from build123d import *

# Parameters (mm, degrees)
F1_DEPTH = 101.6
F2_R     = 5.08
F3_W     = 84.073769
F3_H     = 17.519306
F4_DEPTH = 65.613113


with BuildPart() as f1:
    # F0 (on Right) → F1 (new body)
    with BuildSketch(Plane.YZ):
        Polygon((-46.600301, 33.859685), (-63.820757, 33.859685), (-63.820757, -25.866956), (-42.458672, -25.866956), (-42.458672, -17.365716), (-15.865058, -17.365716), (-15.865058, -26.084935), (1.791356, -26.084935), (1.791356, 3.996365), (-46.600301, 3.996365), align=None)
    extrude(amount=F1_DEPTH)

    # F2
    f2_edges = [f1.edges().sort_by_distance(p)[0] for p in [
        (50.8, -63.820757, 33.859685),
        (50.8, -63.820757, -25.866956),
        (0, -63.820757, 3.996365),
        (101.6, -63.820757, 3.996365),
        (50.8, 1.791356, 3.996365),
        (101.6, -22.404472, 3.996365),
        (0, -22.404472, 3.996365),
        (0, -55.210529, 33.859685),
        (50.8, -46.600301, 33.859685),
        (101.6, -55.210529, 33.859685),
        (101.6, -46.600301, 18.928025),
        (0, -46.600301, 18.928025),
    ]]
    fillet(f2_edges, radius=F2_R)

    # F3 (on face) → F4 (cut, through all)
    with BuildSketch(Plane(origin=(0, 1.791356, 0), x_dir=(-1, 0, 0), z_dir=(0, 1, 0))):
        with Locations((-50.707488, -17.325282)):
            Rectangle(F3_W, F3_H)
    extrude(amount=-F4_DEPTH, mode=Mode.SUBTRACT)


solid = f1.part
Model file for the job. Use its own axes, mm. A direction names the side the tool comes from. Coordinates: 2 decimals unless noted, no trailing zeros. Order: outer loops, then holes, each group sorted by start corner. A loop starts at its lowest first (then second) coordinate and runs counter-clockwise, first axis right, second up. Notation, with made-up numbers: (-15.75, 55) -> (4.25, 55) arc R10 cw to (4.25, 67) -> close; hole circle Ø9 at (19.5, 76). An arc over 180 degrees is marked (long way). Return JSON: item names as keys, results as strings. Group by question number.
Item 1: Saw through at A-A on z = -15. Write the cut outline in (x, y).
Item 2: Saw through at D-D on y = -6. Write the cut outline in (x, z).
Item 3: Saw through at C-C on y = -38.5. Write the cut outline in (x, z).
Item 4: Pull direction Y, two halves, no side cores. Call faces 6 (the cylindrical face through (100.07, -25.32, 2.55)), 7 (the cylindrical face through (100.072, -62.372, 1.074)), 8 (the flat face through (97, -42.459, -22)), 9 (the cylindrical face through (100.072, -48.049, 14.057)): pulls with the +Y half, pulls with the -Y half, needs draft (parallel to the pull), parting line crosses it, or undercut.
Item 5: Tool access for faces 1 (the flat face through (92.744, -31, -16)), 2 (the flat face through (4, -51, -25.867)), 3 (the flat face through (50, -46.6, 16)), 4 (the cylindrical face through (1.528, -48.049, 14.057)), 5 (the flat face through (50, -63.821, 10)): list every direction of +Z, -Z, +X, -X, +Y, -Y with a clear straight run to the whole face (end or side of a thin tool).
Item 6: Saw through at B-B on x = 68.5. Write the cut outline in (y, z), then the cut area to 3 significant figures.
Item 7: Flat gauge pins, fed straight in: P1, Ø9.5, axis at x = 97.5, y = -48, coming from the -Z side; P2, Ø7, axis at x = 97, y = -28.5, coming from the -Z side; P3, Ø19.5, axis at x = 47.5, y = -16, coming from the -Z side. Where does each tip first touch, or does it go through?
Item 8: Wall check: line 1 along X through (y, z) = (-51.5, -9); line 2 along Y through (x, z) = (95, 4.5); line 3 along Z through (x, y) = (6, -53). Give the ranges that are in metal, low to high. Write a range as [from, to].
Values found:
{
 "1": {"outline": "(0, -58.74) arc R5.08 ccw to (5.08, -63.82) -> (8.67, -63.82) -> (8.67, 1.79) -> (0, 1.79) -> close; (92.74, -63.82) -> (96.52, -63.82) arc R5.08 ccw to (101.6, -58.74) -> (101.6, 1.79) -> (92.74, 1.79) -> close"},
 "2": {"outline": "(0, -26.08) -> (8.67, -26.08) -> (8.67, -8.57) -> (92.74, -8.57) -> (92.74, -26.08) -> (101.6, -26.08) -> (101.6, -1.08) arc R5.08 ccw to (96.52, 4) -> (5.08, 4) arc R5.08 ccw to (0, -1.08) -> close"},
 "3": {"outline": "(0, -17.37) -> (8.67, -17.37) -> (8.67, -8.57) -> (92.74, -8.57) -> (92.74, -17.37) -> (101.6, -17.37) -> (101.6, -1.08) arc R5.08 ccw to (96.52, 4) -> (5.08, 4) arc R5.08 ccw to (0, -1.08) -> close"},
 "4": {"face 6": "needs draft", "face 7": "pulls with the -Y half", "face 8": "undercut", "face 9": "pulls with the +Y half"},
 "5": {"face 1": "-Z, +Y, -Y", "face 2": "-Z, +X, -X, -Y", "face 3": "+Z, +X, -X, +Y", "face 4": "+Z, -X, +Y", "face 5": "+Z, -Z, +X, -X, -Y"},
 "6": {"outline": "(-63.82, -8.57) -> (1.79, -8.57) -> (1.79, -1.08) arc R5.08 ccw to (-3.29, 4) -> (-46.6, 4) -> (-46.6, 28.78) arc R5.08 ccw to (-51.68, 33.86) -> (-58.74, 33.86) arc R5.08 ccw to (-63.82, 28.78) -> close", "area": "1,320 mm2"},
 "7": {"P1": "stops at z = -25.87", "P2": "stops at z = -17.37", "P3": "stops at z = -8.57"},
 "8": {"line 1": "x = [0, 8.67], [92.74, 101.6]", "line 2": "y = [-63.82, -46.6]", "line 3": "z = [-25.87, 33.86]"}
}
